```python
from build123d import *

# Parameters (mm, degrees)
F2_DEPTH = 4
F0_R     = 11.5
F3_DEPTH = 4


with BuildPart() as f2:
    # F1 (on Top) → F2 (new body, symmetric)
    with BuildSketch(Plane.XY):
        with BuildLine():
            Line((-12.4521264806, 25.5733730193), (-12.4521264806, 28.0924))
            Line((-12.4521264806, 28.0924), (-6.1021264806, 28.0924))
            Line((-6.1021264806, 28.0924), (-6.1021264806, 16.9323248421))
            ThreePointArc((-6.1021264806, 16.9323248421), (6.472750331, 17.143546912), (12.7, 28.0702803284))
            ThreePointArc((12.7, 28.0702803284), (-1.2545903108, 40.7081600221), (-12.4521264806, 25.5733730193))
        make_face()
        with BuildLine():
            Line((-6.1021264806, 28.0924), (-12.4521264806, 28.0924))
            Line((-12.4521264806, 28.0924), (-12.4521264806, 25.5733730193))
            ThreePointArc((-12.4521264806, 25.5733730193), (-10.2338655521, 20.5497753013), (-6.1021264806, 16.9323248421))
            Line((-6.1021264806, 16.9323248421), (-6.1021264806, 28.0924))
        make_face()
        with BuildLine():
            ThreePointArc((-6.1021264806, 16.9323248421), (-10.2338655521, 20.5497753013), (-12.4521264806, 25.5733730193))
            Line((-12.4521264806, 25.5733730193), (-12.4521264806, 2.4969073091))
            ThreePointArc((-12.4521264806, 2.4969073091), (-10.2338655521, 7.5205050271), (-6.1021264806, 11.1379554863))
            Line((-6.1021264806, 11.1379554863), (-6.1021264806, 16.9323248421))
        make_face()
        with BuildLine():
            ThreePointArc((-6.1021264806, 11.1379554863), (-10.2338655521, 7.5205050271), (-12.4521264806, 2.4969073091))
            Line((-12.4521264806, 2.4969073091), (-12.4521264806, 0))
            Line((-12.4521264806, 0), (-6.1021264806, 0))
            Line((-6.1021264806, 0), (-6.1021264806, 11.1379554863))
        make_face()
        with BuildLine():
            Line((-12.4521264806, 0), (-12.4521264806, 2.4969073091))
            ThreePointArc((-12.4521264806, 2.4969073091), (-7.5233189099, -10.2317971335), (6.096, -11.1413097973))
            Line((6.096, -11.1413097973), (6.096, 0))
            Line((6.096, 0), (12.446, 0))
            Line((12.446, 0), (12.446, -2.5272680903))
            ThreePointArc((12.446, -2.5272680903), (12.6363404513, -1.27), (12.7, 0))
            ThreePointArc((12.7, 0), (6.472750331, 10.9267334164), (-6.1021264806, 11.1379554863))
            Line((-6.1021264806, 11.1379554863), (-6.1021264806, 0))
            Line((-6.1021264806, 0), (-12.4521264806, 0))
        make_face()
        with BuildLine():
            ThreePointArc((12.446, -2.5272680903), (10.2226155965, -7.535789963), (6.096, -11.1413097973))
            Line((6.096, -11.1413097973), (6.096, -16.9388947044))
            ThreePointArc((6.096, -16.9388947044), (10.2226155965, -20.5444145387), (12.446, -25.5529364115))
            Line((12.446, -25.5529364115), (12.446, -2.5272680903))
        make_face()
        with BuildLine():
            Line((6.096, 0), (6.096, -11.1413097973))
            ThreePointArc((6.096, -11.1413097973), (10.2226155965, -7.535789963), (12.446, -2.5272680903))
            Line((12.446, -2.5272680903), (12.446, 0))
            Line((12.446, 0), (6.096, 0))
        make_face()
        with BuildLine():
            ThreePointArc((12.446, -25.5529364115), (10.2226155965, -20.5444145387), (6.096, -16.9388947044))
            Line((6.096, -16.9388947044), (6.096, -28.0924))
            Line((6.096, -28.0924), (12.446, -28.0924))
            Line((12.446, -28.0924), (12.446, -25.5529364115))
        make_face()
        with BuildLine():
            Line((6.096, -28.0924), (6.096, -16.9388947044))
            ThreePointArc((6.096, -16.9388947044), (-10.9249530891, -34.555959284), (12.7, -28.0802045017))
            ThreePointArc((12.7, -28.0802045017), (12.6363404513, -26.8102045017), (12.446, -25.5529364115))
            Line((12.446, -25.5529364115), (12.446, -28.0924))
            Line((12.446, -28.0924), (6.096, -28.0924))
        make_face()
    extrude(amount=F2_DEPTH, both=True)

    # F0 (on Top) → F3 (cut, symmetric)
    with BuildSketch(Plane.XY):
        Circle(F0_R)
        with Locations((0, 28.08)):
            Circle(F0_R)
        with Locations((0, -28.08)):
            Circle(F0_R)
    extrude(amount=F3_DEPTH, both=True, mode=Mode.SUBTRACT)


solid = f2.part
```
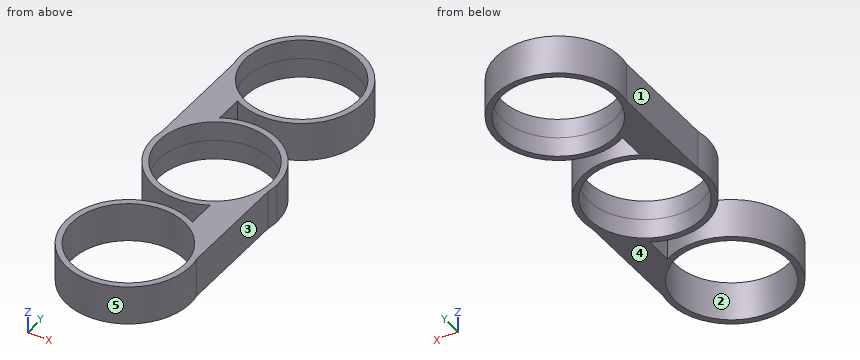
Build history of the part. All positions in model axes, mm. Face numbers are marked on the shaded views. A direction names the side the tool comes from. Give positions to 0.01 mm unless a question says otherwise; leave off trailing zeros. Order: outer loops, then holes, each group sorted by start corner. A loop starts at its lowest first (then second) coordinate and runs counter-clockwise, first axis right, second up. Notation, with made-up numbers: M -4.5,-13 L -0.5,-13 A24 cw -0.5,12 Z; hole C 21,-10 d1. An arc over 180 degrees is marked long. Return JSON: item names as keys, results as strings.
Q1. Wall check: probe 1 along Y at (x, z) = (0, 2.65); probe 2 along Y at (x, z) = (7.5, -2.25); probe 3 along Y at (x, z) = (7.75, 1.5). Give the ranges that are in metal, low to high. Write a range as from..to.
Answer list:
{"probe 1": "y = -40.78..-39.58, -16.58..-15.38, -12.7..-11.5, 11.5..12.7, 15.37..16.58, 39.58..40.77", "probe 2": "y = -38.33..-36.8, -19.36..-8.72, 8.72..10.25, 17.82..19.36, 36.8..38.32", "probe 3": "y = -38.14..-36.58, -19.58..-8.5, 8.5..10.06, 18.01..19.58, 36.58..38.13"}
Q2. Band-saw the part on D-D (x = -7). Give the cut face in (y, z), then the cut area to 3 significant figures.
Answer list:
{"outline": "M -38.68,-4 L -37.2,-4 L -37.2,4 L -38.68,4 Z; M -18.96,-4 L -17.48,-4 L -17.48,4 L -18.96,4 Z; M -10.6,-4 L -9.12,-4 L -9.12,4 L -10.6,4 Z; M 9.12,-4 L 18.96,-4 L 18.96,4 L 9.12,4 Z; M 37.2,-4 L 38.67,-4 L 38.67,4 L 37.2,4 Z", "area": "126 mm^2"}
Q3. Flat gauge pins, fed straight in: pin 1 (1.5 mm diameter, centred on y = 4.5, z = -2.5, fed in from -X); pin 2 (4 mm diameter, centred on x = 7.5, z = -2.5, fed in from -Y). Where does each tip first touch, or does it go through?
Answer list:
{"pin 1": "stops at x = -12.45", "pin 2": "stops at y = -39.53"}
Q4. Band-saw the part on C-C (x = 8.25). Give the cut face in (y, z).
Answer list:
{"outline": "M -37.74,-4 L -36.09,-4 L -36.09,4 L -37.74,4 Z; M -20.07,-4 L -8.01,-4 L -8.01,4 L -20.07,4 Z; M 8.01,-4 L 9.66,-4 L 9.66,4 L 8.01,4 Z; M 18.41,-4 L 20.07,-4 L 20.07,4 L 18.41,4 Z; M 36.09,-4 L 37.73,-4 L 37.73,4 L 36.09,4 Z"}
Q5. 3-axis set-ups, long thin cutter, end or side, ignore diameter. For the marked faces 1, 2 and 3: which of +Z, -Z, +X, -X, +Y, -Y reach the whole face in a straight line?
Answer list:
{"face 1": "+Z, -Z, -X", "face 2": "+Z, -Z", "face 3": "+Z, -Z, +X"}
Q6. Two-plate mould, pull along Y, no slides. Class the marked faces 4 and 5: pulls with the +Y half, pulls with the -Y half, needs draft (parallel to the pull), parting line crosses it, or undercut.
Answer list:
{"face 4": "needs draft", "face 5": "undercut"}
Q7. Band-saw the part on B-B (z = -1). Give the cut face in (x, y), then the cut area to 3 significant figures.
Answer list:
{"outline": "M -12.45,2.5 A12.7 ccw 6.1,-11.14 L 6.1,-16.94 A12.7 ccw long 12.45,-25.55 L 12.45,-2.53 A12.7 ccw -6.1,11.14 L -6.1,16.93 A12.7 ccw long -12.45,25.57 Z; hole C 0,-28.08 d23; hole C 0,0 d23; hole C 0,28.08 d23", "area": "423 mm^2"}
Q8. Band-saw the part on A-A (x = 0). Give the cut face in (y, z), then the cut area to 3 significant figures.
Answer list:
{"outline": "M -40.78,-4 L -39.58,-4 L -39.58,4 L -40.78,4 Z; M -16.58,-4 L -15.38,-4 L -15.38,4 L -16.58,4 Z; M -12.7,-4 L -11.5,-4 L -11.5,4 L -12.7,4 Z; M 11.5,-4 L 12.7,-4 L 12.7,4 L 11.5,4 Z; M 15.37,-4 L 16.58,-4 L 16.58,4 L 15.37,4 Z; M 39.58,-4 L 40.77,-4 L 40.77,4 L 39.58,4 Z", "area": "57.6 mm^2"}
